Design review of the part built by this model. Coordinates are the model's own, in mm. Coordinates: 2 decimals unless noted, no trailing zeros. Loops run counter-clockwise (first coordinate to the right, second up) from the corner with the lowest first, then second, coordinate; pieces in that order, holes last. Notation, with made-up numbers: (-9.75, 47) - (8.25, 47) arc R32 ccw to (8.25, 77) - close; hole circle Ø4 at (53.25, -15.5). An arc over 180 degrees is marked (long way). Use one line per item in the form item = value. Start each with the question number.
(1) Add section D-D (x = -18.15). State the section outline as (y, z) points (3 decimals).
(2) The part is to be moulded in two halves that separate along X. For faces 1 (the face through (40.05, 0, 0)), 2 (the face through (-34.54, 0.27, 0.89)), 3 (the face through (-1, -6.43, 0)), say which applies: pulls with the +X half, pulls with the -X half, needs draft (parallel to the pull), parting line crosses it, or undercut.
(3) Add section C-C (z = 0). Count the separate pieces of the cut face and the enclosed holes in it, plus the area to 3 significant figures.
(4) Add section B-B (x = -3.3). State the section outline as (y, z) points.
(5) For L1, parallel to Z at x = 33.15, y = 3.25; L2, parallel to X at y = 1.5, z = 0; L3, parallel to Y at x = -3.3, z = 3.5, list the stretches that pass through material, from the lowest coordinate up.
(6) Add section A-A (y = 0). State the section outline as (x, z) points, plus the area to 3 significant figures.
(7) Clearance check with a flat-ended pin moving along its axis: pin 1 Ø6 at (x, y) = (-3.3, 0) entering from +Z. State where the tip first meets the part, or that it passes through.
```python
from build123d import *

# Parameters (mm, degrees)
IZIM1_W                     = 80.1
IZIM1_H                     = 12.86
Y_KSEKLIK_EKSTR_ZYON2_DEPTH = 6.43
M4_TAPPED_HOLE1_AT_2_COUNT  = 2
M4_TAPPED_HOLE1_AT_2_PITCH  = 15
M4_TAPPED_HOLE1_AT_3_COUNT  = 2
M4_TAPPED_HOLE1_AT_3_PITCH  = 51.3
M4_TAPPED_HOLE1_AT_4_COUNT  = 2
M4_TAPPED_HOLE1_AT_4_PITCH  = 66.3


with BuildPart() as part:
    # Çizim1 → Yükseklik-Ekstrüzyon2 (new body, symmetric)
    with BuildSketch(Plane.XY):
        Rectangle(IZIM1_W, IZIM1_H)
        with BuildLine():
            ThreePointArc((0, 3.756327994), (-8.3, 0), (0, -3.756327994))
            ThreePointArc((0, -3.756327994), (8.3, 0), (0, 3.756327994))
        make_face(mode=Mode.SUBTRACT)
    extrude(amount=Y_KSEKLIK_EKSTR_ZYON2_DEPTH, both=True)

    # Çizim8 → M4 Tapped Hole1 (revolve, cut)
    with BuildSketch(Plane(origin=(-33.15, 6.43, 0), x_dir=(0, 0, 1), z_dir=(1, 0, 0))):
        Polygon((0, 0), (0, 12.86), (2.025, 12.86), (1.65, 12.485), (1.65, 0), align=None)
    m4_tapped_hole1 = revolve(axis=Axis((-33.15, 12.78, 0), (0, -1, 0)), mode=Mode.SUBTRACT)

    # M4 Tapped Hole1 at 2: M4 Tapped Hole1 ×2
    with Locations(*[(i * M4_TAPPED_HOLE1_AT_2_PITCH, 0, 0) for i in range(1, M4_TAPPED_HOLE1_AT_2_COUNT)]):
        add(m4_tapped_hole1, mode=Mode.SUBTRACT)

    # M4 Tapped Hole1 at 3: M4 Tapped Hole1 ×2
    with Locations(*[(i * M4_TAPPED_HOLE1_AT_3_PITCH, 0, 0) for i in range(1, M4_TAPPED_HOLE1_AT_3_COUNT)]):
        add(m4_tapped_hole1, mode=Mode.SUBTRACT)

    # M4 Tapped Hole1 at 4: M4 Tapped Hole1 ×2
    with Locations(*[(i * M4_TAPPED_HOLE1_AT_4_PITCH, 0, 0) for i in range(1, M4_TAPPED_HOLE1_AT_4_COUNT)]):
        add(m4_tapped_hole1, mode=Mode.SUBTRACT)


solid = part.part
```
Computed values:
q1.outline = (-6.43, -6.43) - (6.43, -6.43) - (6.43, -1.65) - (-6.055, -1.65) - (-6.43, -2.025) - close; (-6.43, 2.025) - (-6.055, 1.65) - (6.43, 1.65) - (6.43, 6.43) - (-6.43, 6.43) - close
q2.face_1 = pulls with the +X half
q2.face_2 = undercut
q2.face_3 = needs draft
q3.separate_pieces = 5
q3.enclosed_holes = 1
q3.area = 720 mm^2
q4.outline = (-6.43, -6.43) - (-5, -6.43) - (-5, 6.43) - (-6.43, 6.43) - close; (5, -6.43) - (6.43, -6.43) - (6.43, 6.43) - (5, 6.43) - close
q5.L1 = -6.43 to -1.65, 1.65 to 6.43
q5.L2 = -40.05 to -34.8, -31.5 to -19.8, -16.5 to -8.07, 8.07 to 16.5, 19.8 to 31.5, 34.8 to 40.05
q5.L3 = -6.43 to -5, 5 to 6.43
q6.outline = (-40.05, -6.43) - (-8.3, -6.43) - (-8.3, 6.43) - (-40.05, 6.43) - close; (8.3, -6.43) - (40.05, -6.43) - (40.05, 6.43) - (8.3, 6.43) - close; hole circle Ø3.3 at (-33.15, 0); hole circle Ø3.3 at (-18.15, 0); hole circle Ø3.3 at (18.15, 0); hole circle Ø3.3 at (33.15, 0)
q6.area = 782 mm^2
q7.pin_1 = through
